```python
from build123d import *

# Parameters (mm, degrees)
SKETCH_1_W          = 40.5
SKETCH_1_H          = 40.5
EXTRUDE_1_DEPTH     = 20
SKETCH_2_R          = 6.5
EXTRUDE_2_DEPTH     = 1.5
SKETCH_5_R          = 0.75
CUT_EXTRUDE_1_DEPTH = 50.500631309
SKETCH_12_R         = 3
EXTRUDE_3_DEPTH     = 4
CHAMFER_1_SIZE2     = 0.545955351
CHAMFER_1_SIZE      = 1.5
CHAMFER_2_SIZE      = 0.5
EXTRUDE_START       = 1.5
SKETCH_18_R         = 3
SKETCH_18_R_2       = 1.25
EXTRUDE_4_DEPTH     = 1.5
FILLET_2_R          = 1
FILLET_3_R          = 1


with BuildPart() as part:
    # 草圖1 → 伸長1 (new body)
    with BuildSketch(Plane.XY):
        Rectangle(SKETCH_1_W, SKETCH_1_H)
    extrude(amount=EXTRUDE_1_DEPTH)

    # 草圖2 → 伸長2 (add)
    with BuildSketch(Plane(origin=(0, 20.25, 0), x_dir=(1, 0, 0), z_dir=(0, 1, 0))):
        with Locations(Location((-9.75, -10, 0), (0, 0, 90))):
            Circle(SKETCH_2_R)
    extrude(amount=EXTRUDE_2_DEPTH)

    # 草圖5 → 除料-伸長1 (cut, through all)
    with BuildSketch(Plane(origin=(0, 20.25, 0), x_dir=(1, 0, 0), z_dir=(0, 1, 0))):
        with Locations(Location((-17.5, -2.5, 0), (0, 0, 270))):
            Circle(SKETCH_5_R)
        with Locations(Location((0, -2.5, 0), (0, 0, 270))):
            Circle(SKETCH_5_R)
        with Locations(Location((17.5, -2.5, 0), (0, 0, 270))):
            Circle(SKETCH_5_R)
        with Locations(Location((17.5, -17.5, 0), (0, 0, 90))):
            Circle(SKETCH_5_R)
        with Locations(Location((0, -17.5, 0), (0, 0, 90))):
            Circle(SKETCH_5_R)
        with Locations(Location((-17.5, -17.5, 0), (0, 0, 90))):
            Circle(SKETCH_5_R)
    extrude(amount=-CUT_EXTRUDE_1_DEPTH, mode=Mode.SUBTRACT)

    # 草圖12 → 伸長3 (add)
    with BuildSketch(Plane(origin=(0, 21.75, 0), x_dir=(1, 0, 0), z_dir=(0, 1, 0))):
        with Locations(Location((-9.75, -10, 0), (0, 0, 270))):
            Circle(SKETCH_12_R)
    extrude(amount=EXTRUDE_3_DEPTH)

    # 導角1
    chamfer_1_edges = [part.edges().sort_by_distance(p)[0] for p in [
        (-9.75, 21.75, 16.5),
    ]]
    chamfer_1_side = [part.faces().sort_by_distance(p)[0] for p in [
        (-9.75, 21.739080893, 16.5),
    ]]
    chamfer(chamfer_1_edges, length=CHAMFER_1_SIZE - 0.0001, length2=CHAMFER_1_SIZE2 - 0.0001, reference=chamfer_1_side[0])  # a hair under: the kernel refuses the full size

    # 導角2
    chamfer_2_edges = [part.edges().sort_by_distance(p)[0] for p in [
        (-9.75, 25.75, 7),
    ]]
    chamfer(chamfer_2_edges, length=CHAMFER_2_SIZE)

    # 草圖18 → 伸長4 (add)
    with BuildSketch(Plane.XZ.offset(20.25).offset(EXTRUDE_START)):
        with Locations(Location((-9.75, 10, 0), (0, 0, 90))):
            Circle(SKETCH_18_R)
        with Locations(Location((-9.75, 10, 0), (0, 0, 270))):
            Circle(SKETCH_18_R_2, mode=Mode.SUBTRACT)
    extrude(amount=-EXTRUDE_4_DEPTH)

    # 圓角2
    fillet_2_edges = [part.edges().sort_by_distance(p)[0] for p in [
        (20.25, 0, 20),
        (-20.25, 0, 20),
        (20.25, 0, 0),
        (-20.25, 0, 0),
    ]]
    fillet(fillet_2_edges, radius=FILLET_2_R)

    # 圓角3
    fillet_3_edges = [part.edges().sort_by_distance(p)[0] for p in [
        (0, -20.25, 20),
        (0, 20.25, 20),
        (0, 20.25, 0),
        (-20.25, 20.25, 10),
        (20.25, 20.25, 10),
        (-19.957106781, 20.25, 19.707106781),
        (-19.957106781, 20.25, 0.292893219),
        (19.957106781, 20.25, 0.292893219),
        (19.957106781, 20.25, 19.707106781),
        (20.25, -20.25, 10),
        (0, -20.25, 0),
        (-20.25, -20.25, 10),
        (-19.957106781, -20.25, 19.707106781),
        (-19.957106781, -20.25, 0.292893219),
        (19.957106781, -20.25, 0.292893219),
        (19.957106781, -20.25, 19.707106781),
    ]]
    fillet(fillet_3_edges, radius=FILLET_3_R)


solid = part.part
```
Could you check a few things on this model? Use its own coordinates, in mm. A direction names the side the tool comes from. Coordinates: 2 decimals unless noted, no trailing zeros. Write each loop counter-clockwise with the first axis right and the second up, starting at its lowest first coordinate (ties: lowest second). Pieces come first, ordered by that corner, then holes. Notation, with made-up numbers: (3, 75) -> (21, 75) arc R29 cw to (21, 114) -> close; hole circle Ø10 at (42.25, 85). An arc over 180 degrees is marked (long way). Write item = value, one per line. Start each with the question number.
(1) Which directions (+Z, -Z, +X, -X, +Y, -Y) give clear straight access to the entire face, cutting with the end or side of a thin tool? Please do faces 5 (the face through (-0.27, -19.949, 0.285)), 6 (the face through (-11, 21.75, 13)), 7 (the face through (-10, -20.25, 10)).
(2) I want a section at C-C (x = 2). Please give me the cut outline in (y, z).
(3) We'd pull the mould along Z, two halves only. Please class faces 1 (the face through (0.456, 0.284, 18.095)), 2 (the face through (19.949, 0.27, 19.715)), 3 (the face through (19.965, -19.949, 9.874)), 4 (the face through (-0.27, 19.965, 0.301)): released by +Z, released by -Z, zero draft, split by the parting line, or undercut.
(4) Will these pins go through, and if not, where does the flat tip stop? pin 1 (12 mm diameter, centred on x = -2, z = 15.5, fed in from +Y); pin 2 (9 mm diameter, centred on x = -1.5, z = 6, fed in from -Y); pin 3 (1 mm diameter, centred on x = 16, z = 6.5, fed in from +Y).
(5) I need wall thicknesses on line 1 (X direction, y = 9, z = 17.5); line 2 (Z direction, x = -18, y = -6.5); line 3 (X direction, y = -20.9, z = 10). Which ranges of each line are inside material? Lowest first, please. Write a range as [from, to].
(6) I want a section at B-B (x = -17.5). Please give me the cut outline in (y, z).
(7) I want a section at A-A (z = 2.5). Please give me the cut outline in (x, y).
Result set:
q1.face_5 = -Z, +X, -X, -Y
q1.face_6 = +Y
q1.face_7 = -Y
q2.outline = (-20.25, 1) arc R1 ccw to (-19.25, 0) -> (19.25, 0) arc R1 ccw to (20.25, 1) -> (20.25, 19) arc R1 ccw to (19.25, 20) -> (-19.25, 20) arc R1 ccw to (-20.25, 19) -> close
q3.face_1 = undercut
q3.face_2 = released by +Z
q3.face_3 = zero draft
q3.face_4 = released by -Z
q4.pin_1 = 21.75
q4.pin_2 = -20.25
q4.pin_3 = 20.25
q5.line_1 = [-20.25, -18.25], [-16.75, -0.75], [0.75, 16.75], [18.25, 20.25]
q5.line_2 = [0, 1.94], [3.06, 16.94], [18.06, 20]
q5.line_3 = [-12.75, -11], [-8.5, -6.75]
q6.outline = (-20.25, 1) arc R1 ccw to (-19.25, 0) -> (19.25, 0) arc R1 ccw to (20.25, 1) -> (20.25, 1.75) -> (-20.25, 1.75) -> close; (-20.25, 3.25) -> (20.25, 3.25) -> (20.25, 16.75) -> (-20.25, 16.75) -> close; (-20.25, 18.25) -> (20.25, 18.25) -> (20.25, 19) arc R1 ccw to (19.25, 20) -> (-19.25, 20) arc R1 ccw to (-20.25, 19) -> close
q7.outline = (-20.25, -19.25) arc R1 ccw to (-19.25, -20.25) -> (-18.25, -20.25) -> (-18.25, 20.25) -> (-19.25, 20.25) arc R1 ccw to (-20.25, 19.25) -> close; (-16.75, -20.25) -> (-0.75, -20.25) -> (-0.75, 20.25) -> (-16.75, 20.25) -> close; (0.75, -20.25) -> (16.75, -20.25) -> (16.75, 20.25) -> (0.75, 20.25) -> close; (18.25, -20.25) -> (19.25, -20.25) arc R1 ccw to (20.25, -19.25) -> (20.25, 19.25) arc R1 ccw to (19.25, 20.25) -> (18.25, 20.25) -> close
